Solid Edge part; units mm, degrees
sketch "Sketch1" plane through (0, 0, 0) normal (0, -1, 0) x (1, 0, 0)
  line L0 (-9.4591, 28.4697) -> (-54.4988, 14.3095)
  line L1 (-9.4591, -28.4697) -> (-54.4988, -14.3095)
  arc A0 (-9.4591, 28.4697) -> (-9.4591, -28.4697) centre (0, 0) ccw
  arc A1 (-54.4988, -14.3095) -> (-54.4988, 14.3095) centre (-50, 0) cw
  circle A2 centre (-50, 0) radius 6
extrude "Protrusion1" add sketch "Sketch1" against normal blind 10
sketch "Sketch2" plane through (0, 0, 0) normal (0, -1, 0) x (1, 0, 0)
  line L0 (9.4591, -28.4697) -> (58.9766, -12.0175)
  arc A0 (9.4591, 28.4697) -> (9.4591, -28.4697) centre (0, 0) cw
  line L1 (9.4591, 28.4697) -> (58.9766, 12.0175)
  arc A1 (58.9766, 12.0175) -> (58.9766, -12.0175) centre (50, 0) cw
extrude "ExtrudedProtrusion_2" add sketch "Sketch2" against normal blind 10
sketch "Sketch3" plane through (0, 0, 0) normal (0, -1, 0) x (1, 0, 0)
  circle A0 centre (0, 0) radius 30
extrude "ExtrudedProtrusion_3" add sketch "Sketch3" against normal blind 10
sketch "Sketch4" plane through (0, 0, 0) normal (0, -1, 0) x (1, 0, 0)
  circle A0 centre (0, 0) radius 25
  circle A1 centre (0, 0) radius 10
extrude "ExtrudedProtrusion_6" add sketch "Sketch4" along normal blind 30
sketch "Sketch5" plane through (0, 10, 0) normal (0, 1, 0) x (-0.949, 0, -0.3153)
  circle A0 centre (0, 0) radius 10
extrude "ExtrudedCutout_1" cut sketch "Sketch5" against normal blind 62
sketch "Sketch6" plane through (0, 0, 0) normal (0, -1, 0) x (1, 0, 0)
  circle A0 centre (0, 0) radius 10
  circle A1 centre (0, 0) radius 15
extrude "ExtrudedProtrusion_11" add sketch "Sketch6" against normal blind 20
sketch "Sketch7" plane through (0, 0, 0) normal (0, -1, 0) x (0.954, 0, -0.2999)
  circle A0 centre (47.6982, 14.9961) radius 6
extrude "ExtrudedCutout_2" cut sketch "Sketch7" against normal blind 10
sketch "Sketch8" plane through (0, -30, 0) normal (0, -1, 0) x (0, 0, -1)
  circle A0 centre (0, 0) radius 30
extrude "ExtrudedProtrusion_12" add sketch "Sketch8" along normal blind 12
sketch "Sketch9" plane through (0, -42, 0) normal (0, -1, 0) x (1, 0, 0)
  circle A0 centre (0, 0) radius 20
extrude "ExtrudedCutout_3" cut sketch "Sketch9" against normal blind 42
For this review, take the finished solid that the model builds, in its own axes (mm). A direction names the side the tool comes from. Give positions to 0.01 mm unless a question says otherwise; leave off trailing zeros. Write each loop counter-clockwise with the first axis right and the second up, starting at its lowest first coordinate (ties: lowest second). Pieces come first, ordered by that corner, then holes. Notation, with made-up numbers: M 80.25,-40 L 118.25,-40 A13 cw 118.25,-17 Z; hole C -33.75,2 d7. An arc over 180 degrees is marked long. Answer as a JSON object with one key per item and string values. Group by question number.
Item 1: Consider section D-D on x = -50. Write out the cut boundary in (y, z), plus the area to 3 significant figures.
Item 2: Consider section B-B on z = 2. Count the separate pieces of the cut face and the enclosed holes in it, plus the area to 3 significant figures.
Item 3: Consider section A-A on x = 0. Write out the cut boundary in (y, z), plus the area to 3 significant figures.
Item 4: Consider section C-C on y = -3. Write out the cut boundary in (x, z).
Item 5: For pin 1 Ø12 at (x, z) = (-50.5, -7) entering from +Y; pin 2 Ø15.5 at (x, z) = (-50, 0) entering from -Y; pin 3 Ø20 at (x, z) = (9.5, 3.5) entering from -Y; pin 4 Ø2 at (y, z) = (-24.5, 12) entering from +X, all flat-tipped, find the tip position at first contact; note any pin that passes through.
Item 6: Draft analysis for pull direction Z (two halves, no side actions). For faces 4 (the flat face through (33.87, 4.93, 20.36)), 5 (the flat face through (-28, 0, 0)), 6 (the cylindrical face through (-4.336, -21.294, -19.524)), state which applies: +Z half, -Z half, draft (parallel to the pull), parting line (faces both ways), or undercut.
Item 7: For probe 1 along Z at (x, y) = (0, -20); probe 2 along Z at (x, y) = (0, 16); probe 3 along Y at (x, z) = (41, -17), list the stretches that pass through material, from the lowest coordinate up. Write a range as [from, to].
Item 8: Tool access review of faces 1 (the cylindrical face through (-1.32, -35.92, 29.97)), 2 (the cylindrical face through (-14.985, 14.93, 0.66)), 3 (the flat face through (25, -30, 7)): name each direction out of +Z, -Z, +X, -X, +Y, -Y from which nothing blocks a thin tool from reaching the whole face with its end or side.
Check result:
{
 "1": {"outline": "M 0,-15.72 L 10,-15.72 L 10,-6 L 0,-6 Z; M 0,6 L 10,6 L 10,15.72 L 0,15.72 Z", "area": "194 mm^2"},
 "2": {"separate pieces": "4", "enclosed holes": "0", "area": "1,520 mm^2"},
 "3": {"outline": "M -42,-30 L -30,-30 L -30,-25 L 0,-25 L 0,-30 L 10,-30 L 10,-15 L 20,-15 L 20,-10 L 0,-10 L 0,-20 L -42,-20 Z; M -42,20 L 0,20 L 0,10 L 20,10 L 20,15 L 10,15 L 10,30 L 0,30 L 0,25 L -30,25 L -30,30 L -42,30 Z", "area": "1,040 mm^2"},
 "4": {"outline": "C 0,0 d50; hole C 0,0 d40"},
 "5": {"pin 1": "stops at y = 10", "pin 2": "stops at y = 0", "pin 3": "stops at y = -42", "pin 4": "stops at x = 22.45"},
 "6": {"face 4": "+Z half", "face 5": "draft", "face 6": "undercut"},
 "7": {"probe 1": "z = [-25, -20], [20, 25]", "probe 2": "z = [-15, -10], [10, 15]", "probe 3": "y = [0, 10]"},
 "8": {"face 1": "-Y", "face 2": "+Y", "face 3": "none"}
}
